Model file for the job. Use its own axes, mm. Round coordinates to 2 decimals unless told otherwise and drop trailing zeros. Order: outer loops, then holes, each group sorted by start corner. A loop starts at its lowest first (then second) coordinate and runs counter-clockwise, first axis right, second up. Notation, with made-up numbers: M -17,64.25 L -6,64.25 A23 ccw -6,90.25 Z; hole C 9.5,-16 d1. An arc over 180 degrees is marked long. Return JSON: item names as keys, results as strings. Group by question number.
Item 1: Pull direction X, two halves, no side cores. Call faces 1 (the face through (-3, 4, -271)), 2 (the face through (0, 0, -271)), 3 (the face through (0.2, 3.94, -349.25)): pulls with the +X half, pulls with the -X half, needs draft (parallel to the pull), parting line crosses it, or undercut.
Item 2: Probe line 1 along Z through (x, y) = (0, 3.5) (3 decimals); line 2 along Z through (x, y) = (0.5, 1.25); line 3 along Z through (x, y) = (2.75, 3.5). List the from-to ranges inside material, lowest first.
Item 3: Slice it at A-A on x = 0. Write the cut outline in (y, z) (3 decimals), then the cut area to 3 significant figures.
Autodesk Inventor part; units mm, degrees
ref_plane "YZ Plane" through (0, 0, 0) normal (1, 0, 0) x (0, 1, 0)
ref_plane "XZ Plane" through (0, 0, 0) normal (0, 1, 0) x (-1, 0, 0)
ref_plane "XY Plane" through (0, 0, 0) normal (0, 0, 1) x (1, 0, 0)
sketch "Sketch1" plane through (0, 0, 0) normal (0, 1, 0) x (-1, 0, 0)
  line L0 (0, 0) -> (0, -347.765) construction
  line L1 (-3, 0) -> (-3, -347.765)
  line L2 (3, -347.765) -> (3, 0)
  arc A0 (3, 0) -> (-3, 0) centre (0, 0) ccw
  arc A1 (-3, -347.765) -> (3, -347.765) centre (0, -347.765) ccw
  circle A2 centre (0, 0) radius 1.5
  circle A3 centre (0, -347.765) radius 1.5
  circle A4 centre (0, -131.233) radius 1.5
  circle A5 centre (0, -37.934) radius 1.5
  point P0 (0, -173.8825)
  dimension "d0" = 347.765
  dimension "d1" = 6
  dimension "d2" = 3
  dimension "d3" = 3
  dimension "d6" = 3
  dimension "d7" = 131.233
  dimension "d8" = 3
  dimension "d9" = 37.934
extrude "Extrusion1" add sketch "Sketch1" along normal blind 8
sketch "Sketch2" plane through (0, 8, 0) normal (0, 1, 0) x (1, 0, 0)
  arc A0 (3, 347.765) -> (-3, 347.765) centre (0, 347.765) ccw
  line L0 (-3, 347.765) -> (-3, 0)
  arc A1 (-3, 0) -> (3, 0) centre (0, 0) ccw
  line L1 (3, 0) -> (3, 347.765)
  circle A2 centre (0, 131.233) radius 1.5
  circle A3 centre (0, 37.934) radius 1.5
  circle A4 centre (0, 347.765) radius 1.5
  circle A5 centre (0, 0) radius 1.5
sketch "Sketch3" plane through (0, 8, 0) normal (0, 1, 0) x (1, 0, 0)
  line L0 (-13.5041, 192.6393) -> (33.2898, 192.6393)
  line L1 (33.2898, 192.6393) -> (33.2898, -23.3325)
  line L2 (33.2898, -23.3325) -> (-13.5041, -23.3325)
  line L3 (-13.5041, -23.3325) -> (-13.5041, 192.6393)
  line L4 (-64.7974, 383.8644) -> (82.7834, 383.8644)
  line L5 (82.7834, 383.8644) -> (82.7834, -81.8249)
  line L6 (82.7834, -81.8249) -> (-64.7974, -81.8249)
  line L7 (-64.7974, -81.8249) -> (-64.7974, 383.8644)
  point P0 (0, 0)
extrude "Extrusion2" cut sketch "Sketch3" against normal blind 10 contours L0 L1 L2 L3
sketch "Sketch4" plane through (0, 8, 0) normal (0, 1, 0) x (1, 0, 0)
  line L0 (-3, 192.6393) -> (3, 192.6393)
  line L1 (3, 192.6393) -> (3, 347.765)
  arc A0 (3, 347.765) -> (-3, 347.765) centre (0, 347.765) ccw
  line L2 (-3, 347.765) -> (-3, 192.6393)
  circle A1 centre (0, 347.765) radius 1.5
  point P0 (0, 0)
properties part number "Part_10_p1"
Output values:
{
 "1": {"face 1": "pulls with the -X half", "face 2": "needs draft", "face 3": "undercut"},
 "2": {"line 1": "-350.765 to -349.265, -346.265 to -192.639", "line 2": "-350.72 to -349.18, -346.35 to -192.64", "line 3": "-348.96 to -192.64"},
 "3": {"outline": "M 0,-350.765 L 8,-350.765 L 8,-349.265 L 0,-349.265 Z; M 0,-346.265 L 8,-346.265 L 8,-192.639 L 0,-192.639 Z", "area": "1,240 mm²"}
}
